```python
from build123d import *

# Parameters (mm, degrees)
ESQUISSE1_R             = 107.95
BOSS_EXTRU_1_DEPTH      = 5.588
ESQUISSE2_R             = 1.905
ENL_V_MAT_EXTRU_1_DEPTH = 5.588
ENL_V_MAT_EXTRU_2_DEPTH = 5.588
ESQUISSE5_R             = 1
ENL_V_MAT_EXTRU_3_DEPTH = 153.766589096
ESQUISSE6_R             = 2
ENL_V_MAT_EXTRU_4_DEPTH = 153.766589096
ESQUISSE7_R             = 2
ENL_V_MAT_EXTRU_5_DEPTH = 153.766589096
ESQUISSE8_R             = 1.5
ENL_V_MAT_EXTRU_6_DEPTH = 153.766589096


with BuildPart() as part:
    # Esquisse1 → Boss.-Extru.1 (new body)
    with BuildSketch(Plane(origin=(0, 0, 0), x_dir=(1, 0, 0), z_dir=(0, 1, 0))):
        with Locations(Location((0, 0, 0), (0, 0, 270))):
            Circle(ESQUISSE1_R)
    extrude(amount=BOSS_EXTRU_1_DEPTH)

    # Esquisse2 → Enlèv. mat.-Extru.1 (cut)
    with BuildSketch(Plane(origin=(0, 5.588, 0), x_dir=(1, 0, 0), z_dir=(0, 1, 0))):
        with Locations(Location((26.569931805, 99.16033545, 0), (0, 0, 270))):
            Circle(ESQUISSE2_R)
        with Locations(Location((51.329166667, 88.904724577, 0), (0, 0, 270))):
            Circle(ESQUISSE2_R)
        with Locations(Location((72.590403645, 72.590403645, 0), (0, 0, 270))):
            Circle(ESQUISSE2_R)
        with Locations(Location((88.904724577, 51.329166667, 0), (0, 0, 270))):
            Circle(ESQUISSE2_R)
        with Locations(Location((99.16033545, 26.569931805, 0), (0, 0, 270))):
            Circle(ESQUISSE2_R)
        with Locations(Location((99.16033545, -26.569931805, 0), (0, 0, 270))):
            Circle(ESQUISSE2_R)
        with Locations(Location((88.904724577, -51.329166667, 0), (0, 0, 270))):
            Circle(ESQUISSE2_R)
        with Locations(Location((72.590403645, -72.590403645, 0), (0, 0, 270))):
            Circle(ESQUISSE2_R)
        with Locations(Location((51.329166667, -88.904724577, 0), (0, 0, 270))):
            Circle(ESQUISSE2_R)
        with Locations(Location((26.569931805, -99.16033545, 0), (0, 0, 270))):
            Circle(ESQUISSE2_R)
        with Locations(Location((-26.569931805, -99.16033545, 0), (0, 0, 270))):
            Circle(ESQUISSE2_R)
        with Locations(Location((-51.329166667, -88.904724577, 0), (0, 0, 270))):
            Circle(ESQUISSE2_R)
        with Locations(Location((-72.590403645, -72.590403645, 0), (0, 0, 270))):
            Circle(ESQUISSE2_R)
        with Locations(Location((-88.904724577, -51.329166667, 0), (0, 0, 270))):
            Circle(ESQUISSE2_R)
        with Locations(Location((-99.16033545, -26.569931805, 0), (0, 0, 270))):
            Circle(ESQUISSE2_R)
        with Locations(Location((-99.16033545, 26.569931805, 0), (0, 0, 270))):
            Circle(ESQUISSE2_R)
        with Locations(Location((-88.904724577, 51.329166667, 0), (0, 0, 270))):
            Circle(ESQUISSE2_R)
        with Locations(Location((-72.590403645, 72.590403645, 0), (0, 0, 270))):
            Circle(ESQUISSE2_R)
        with Locations(Location((-51.329166667, 88.904724577, 0), (0, 0, 270))):
            Circle(ESQUISSE2_R)
        with Locations(Location((-26.569931805, 99.16033545, 0), (0, 0, 270))):
            Circle(ESQUISSE2_R)
    extrude(amount=-ENL_V_MAT_EXTRU_1_DEPTH, mode=Mode.SUBTRACT)

    # Esquisse3 → Enlèv. mat.-Extru.2 (cut)
    with BuildSketch(Plane(origin=(0, 5.588, 0), x_dir=(1, 0, 0), z_dir=(0, 1, 0))):
        with BuildLine():
            Line((-45.085, -52.07), (45.085, -52.07))
            ThreePointArc((45.085, -52.07), (46.881051224, -51.326051224), (47.625, -49.53))
            Line((47.625, -49.53), (47.625, 11.43))
            ThreePointArc((47.625, 11.43), (46.881051224, 13.226051224), (45.085, 13.97))
            Line((45.085, 13.97), (-45.085, 13.97))
            ThreePointArc((-45.085, 13.97), (-46.881051224, 13.226051224), (-47.625, 11.43))
            Line((-47.625, 11.43), (-47.625, -49.53))
            ThreePointArc((-47.625, -49.53), (-46.881051224, -51.326051224), (-45.085, -52.07))
        make_face()
    extrude(amount=-ENL_V_MAT_EXTRU_2_DEPTH, mode=Mode.SUBTRACT)

    # Esquisse5 → Enlèv. mat.-Extru.3 (cut, through all)
    with BuildSketch(Plane(origin=(0, 5.588, 0), x_dir=(1, 0, 0), z_dir=(0, 1, 0))):
        with Locations(Location((-3.5, -98.95, 0), (0, 0, 270))):
            Circle(ESQUISSE5_R)
        with Locations(Location((3.5, -98.95, 0), (0, 0, 90))):
            Circle(ESQUISSE5_R)
        with Locations(Location((-98.95, 2.5, 0), (0, 0, 270))):
            Circle(ESQUISSE5_R)
        with Locations(Location((-98.95, -4.5, 0), (0, 0, 90))):
            Circle(ESQUISSE5_R)
        with Locations(Location((2.5, 97.95, 0), (0, 0, 270))):
            Circle(ESQUISSE5_R)
        with Locations(Location((-4.5, 97.95, 0), (0, 0, 90))):
            Circle(ESQUISSE5_R)
        with Locations(Location((97.95, -3.5, 0), (0, 0, 270))):
            Circle(ESQUISSE5_R)
        with Locations(Location((97.95, 3.5, 0), (0, 0, 90))):
            Circle(ESQUISSE5_R)
    extrude(amount=-ENL_V_MAT_EXTRU_3_DEPTH, mode=Mode.SUBTRACT)

    # Esquisse6 → Enlèv. mat.-Extru.4 (cut, through all)
    with BuildSketch(Plane(origin=(0, 5.588, 0), x_dir=(1, 0, 0), z_dir=(0, 1, 0))):
        with Locations(Location((-22, -70.07, 0), (0, 0, 270))):
            Circle(ESQUISSE6_R)
        with Locations(Location((22, -70.07, 0), (0, 0, 270))):
            Circle(ESQUISSE6_R)
        with Locations(Location((-22.3, 69.97, 0), (0, 0, 270))):
            Circle(ESQUISSE6_R)
        with Locations(Location((22.3, 69.97, 0), (0, 0, 90))):
            Circle(ESQUISSE6_R)
        with Locations(Location((-58.95, 77.5, 0), (0, 0, 270))):
            Circle(ESQUISSE6_R)
        with Locations(Location((58.95, 77.5, 0), (0, 0, 90))):
            Circle(ESQUISSE6_R)
        with Locations(Location((-22.3, 26.97, 0), (0, 0, 270))):
            Circle(ESQUISSE6_R)
        with Locations(Location((22.15, 26.97, 0), (0, 0, 270))):
            Circle(ESQUISSE6_R)
    extrude(amount=-ENL_V_MAT_EXTRU_4_DEPTH, mode=Mode.SUBTRACT)

    # Esquisse7 → Enlèv. mat.-Extru.5 (cut, through all)
    with BuildSketch(Plane(origin=(0, 5.588, 0), x_dir=(1, 0, 0), z_dir=(0, 1, 0))):
        with Locations(Location((58.881051224, 16.726051224, 0), (0, 0, 270))):
            Circle(ESQUISSE7_R)
        with Locations(Location((-58.881051224, 16.726051224, 0), (0, 0, 90))):
            Circle(ESQUISSE7_R)
    extrude(amount=-ENL_V_MAT_EXTRU_5_DEPTH, mode=Mode.SUBTRACT)

    # Esquisse8 → Enlèv. mat.-Extru.6 (cut, through all)
    with BuildSketch(Plane(origin=(0, 5.588, 0), x_dir=(1, 0, 0), z_dir=(0, 1, 0))):
        with Locations(Location((0, -82.95, 0), (0, 0, 270))):
            Circle(ESQUISSE8_R)
    extrude(amount=-ENL_V_MAT_EXTRU_6_DEPTH, mode=Mode.SUBTRACT)


solid = part.part
```
Model file for the job. Use its own axes, mm. A direction names the side the tool comes from. Round coordinates to 2 decimals unless told otherwise and drop trailing zeros. Write each loop counter-clockwise with the first axis right and the second up, starting at its lowest first coordinate (ties: lowest second). Pieces come first, ordered by that corner, then holes. Notation, with made-up numbers: (69, -18) -> (110, -18) arc R13 cw to (110, -5) -> close; hole circle Ø7 at (40.25, -11). An arc over 180 degrees is marked (long way). Answer as CSV lines item,"result".
1. Drill centre lines: line 1 (X direction, y = 4.2, z = -69.97); line 2 (X direction, y = 4.2, z = -97.5); line 3 (X direction, y = 5.1, z = 50). Where is each one in solid material? Low to high.
Resolved:
line 1,"-82.2 to -24.3, -20.3 to 20.3, 24.3 to 82.2"
line 2,"-46.34 to -27.5, -25.64 to -5.39, -3.61 to 1.61, 3.39 to 25.64, 27.5 to 46.34"
line 3,"-95.67 to -90.27, -87.54 to -47.58, 47.58 to 87.54, 90.27 to 95.67"
2. Slice it at B-B, the plane x = -42.5. List the corners of the cut face in (y, z), plus the area to 3 significant figures.
Resolved:
outline,"(0, -99.23) -> (5.59, -99.23) -> (5.59, -13.97) -> (0, -13.97) -> close; (0, 52.07) -> (5.59, 52.07) -> (5.59, 99.23) -> (0, 99.23) -> close"
area,"740 mm²"
3. Slice it at D-D, the plane x = 83. List the corners of the cut face in (y, z).
Resolved:
outline,"(0, -69.02) -> (5.59, -69.02) -> (5.59, 69.02) -> (0, 69.02) -> close"
4. Mould opens along X. For faces 1 (the face through (72.96, 2.75, -79.56)), 2 (the face through (2, 5.588, -26)), 3 (the face through (1, 3, -13.97)) say: +X half, -X half, draft (parallel to the pull), parting line (faces both ways), or undercut.
Resolved:
face 1,"parting line"
face 2,"draft"
face 3,"undercut"
5. Tool access for faces 4 (the face through (2, 0, -26)), 5 (the face through (47.625, 3, 19)): list every direction of +Z, -Z, +X, -X, +Y, -Y with a clear straight run to the whole face (end or side of a thin tool).
Resolved:
face 4,"+Z, -Z, +X, -X, -Y"
face 5,"+Y, -Y"
6. Slice it at A-A, the plane z = 45. List the corners of the cut face in (x, y) (3 decimals).
Resolved:
outline,"(-98.123, 0) -> (-47.625, 0) -> (-47.625, 5.588) -> (-98.123, 5.588) -> close; (47.625, 0) -> (98.123, 0) -> (98.123, 5.588) -> (47.625, 5.588) -> close"
7. Pin check, flat tips, straight feed: pin 1 Ø2.5 at (x, z) = (26.57, -99.16) entering from +Y; pin 2 Ø1 at (x, y) = (48.5, 1) entering from +Z; pin 3 Ø1.5 at (x, y) = (33, 1) entering from -Z; pin 4 Ø3 at (x, y) = (-29, 3.5) entering from +Z. Stop position of each tip, or through.
Resolved:
pin 1,"through"
pin 2,"z = 96.69"
pin 3,"z = -103.02"
pin 4,"z = 104.39"
8. Slice it at C-C, the plane y = 2.2. State how many separate pieces and enclosed holes the cut face has, plus the area to 3 significant figures.
Resolved:
separate pieces,"1"
enclosed holes,"40"
area,"29,900 mm²"
